Part model, mm, in its own coordinate system. A direction names the side the tool comes from. Give positions to 0.01 mm unless a question says otherwise; leave off trailing zeros. Write each loop counter-clockwise with the first axis right and the second up, starting at its lowest first coordinate (ties: lowest second). Pieces come first, ordered by that corner, then holes. Notation, with made-up numbers: M -13,-3.5 L 40,-3.5 A31 cw 40,27.5 Z; hole C 47.25,-23.75 d7. An arc over 180 degrees is marked long. Answer as CSV lines item,"result". Start each with the question number.
Item 1: Band-saw the part on C-C, the plane y = -8.5. List the corners of the cut face in (x, z).
Item 2: Wall check: L1, parallel to X at y = 9.25, z = 15.75; L2, parallel to Y at x = -1, z = 5.5; L3, parallel to Z at x = -0.75, y = -8. Give the ranges that are in metal, low to high. Write a range as from..to.
Item 3: Band-saw the part on B-B, the plane z = 19.75. List the corners of the cut face in (x, y).
Item 4: 3-axis set-ups, long thin cutter, end or side, ignore diameter. For faces 1 (the flat face through (2.4, 0, 8)), 2 (the flat face through (0, -2.4, 20)), 3 (the flat face through (-4, 0, 0)): which of +Z, -Z, +X, -X, +Y, -Y reach the whole face in a straight line?
Item 5: Pin check, flat tip, straight feed: pin 1 (1.4 mm diameter, centred on x = -0.5, y = 6, fed in from -Z). Stop position of the tip, or through.
Item 6: Two-plate mould, pull along Y, no slides. Class faces 4 (the flat face through (0, -13, 11)), 5 (the flat face through (0, 6, 18)), 6 (the flat face through (0, 13, 11)): +Y half, -Y half, draft (parallel to the pull), parting line (faces both ways), or undercut.
Item 7: Band-saw the part on A-A, the plane x = -2. List the corners of the cut face in (y, z), then the cut area to 3 significant figures.
Item 8: Band-saw the part on D-D, the plane z = 5.75. List the corners of the cut face in (x, y).
from build123d import *

# Parameters (mm, degrees)
SKETCH1_W           = 10.8
SKETCH1_H           = 26
SKETCH1_W_2         = 4.8
SKETCH1_H_2         = 20
BOSS_EXTRUDE1_DEPTH = 18
SKETCH2_W           = 10.8
SKETCH2_H           = 26
SKETCH2_W_2         = 4.8
SKETCH2_H_2         = 4.8
BOSS_EXTRUDE2_DEPTH = 4


with BuildPart() as part:
    # Sketch1 → Boss-Extrude1 (new body)
    with BuildSketch(Plane.XY):
        Rectangle(SKETCH1_W, SKETCH1_H)
        Rectangle(SKETCH1_W_2, SKETCH1_H_2, mode=Mode.SUBTRACT)
    extrude(amount=BOSS_EXTRUDE1_DEPTH)

    # Sketch2 → Boss-Extrude2 (add)
    with BuildSketch(Plane.XY.offset(18)):
        Rectangle(SKETCH2_W, SKETCH2_H)
        Rectangle(SKETCH2_W_2, SKETCH2_H_2, mode=Mode.SUBTRACT)
    extrude(amount=BOSS_EXTRUDE2_DEPTH)


solid = part.part
Output:
1,outline,"M -5.4,0 L -2.4,0 L -2.4,18 L 2.4,18 L 2.4,0 L 5.4,0 L 5.4,22 L -5.4,22 Z"
2,L1,"-5.4..-2.4, 2.4..5.4"
2,L2,"-13..-10, 10..13"
2,L3,"18..22"
3,outline,"M -5.4,-13 L 5.4,-13 L 5.4,13 L -5.4,13 Z; hole M -2.4,-2.4 L 2.4,-2.4 L 2.4,2.4 L -2.4,2.4 Z"
4,face 1,"-Z"
4,face 2,"+Z, -Z"
4,face 3,"-Z, +X, -X, +Y, -Y"
5,pin 1,"z = 18"
6,face 4,"-Y half"
6,face 5,"undercut"
6,face 6,"+Y half"
7,outline,"M -13,0 L -10,0 L -10,18 L -2.4,18 L -2.4,22 L -13,22 Z; M 2.4,18 L 10,18 L 10,0 L 13,0 L 13,22 L 2.4,22 Z"
7,area,"193 mm²"
8,outline,"M -5.4,-13 L 5.4,-13 L 5.4,13 L -5.4,13 Z; hole M -2.4,-10 L 2.4,-10 L 2.4,10 L -2.4,10 Z"
